from build123d import *

# Parameters (mm, degrees)
BOSS_EXTRUDE1_DEPTH                                  = 30
CBORE_FOR_M5_HEX_HEAD_BOLT1_D                        = 5.5
CBORE_FOR_M5_HEX_HEAD_BOLT1_CBORE_D                  = 12.238
CBORE_FOR_M5_HEX_HEAD_BOLT1_CBORE_DEPTH              = 3.5
CSK_FOR_M4_COUNTERSUNK_RAISED_HEAD_SCREW_D           = 4.3
CSK_FOR_M4_COUNTERSUNK_RAISED_HEAD_SCREW_CSINK_D     = 9.4
CSK_FOR_M4_COUNTERSUNK_RAISED_HEAD_SCREW_CSINK_ANGLE = 90


with BuildPart() as part:
    # Sketch1 → Boss-Extrude1 (new body)
    with BuildSketch(Plane.XY):
        Polygon((0, 0), (0, 40), (120, 40), (120, 30), (10, 30), (10, 0), align=None)
    extrude(amount=BOSS_EXTRUDE1_DEPTH)

    # CBORE for M5 Hex Head Bolt1 (through all)
    with Locations(Plane(origin=(0, 30, 0), x_dir=(-1, 0, 0), z_dir=(0, -1, 0))):
        with Locations((-108, -15.41009868), (-28, -15.41009868)):
            CounterBoreHole(CBORE_FOR_M5_HEX_HEAD_BOLT1_D / 2, CBORE_FOR_M5_HEX_HEAD_BOLT1_CBORE_D / 2, CBORE_FOR_M5_HEX_HEAD_BOLT1_CBORE_DEPTH)

    # CSK for M4 Countersunk Raised Head Screw1 (through all)
    with Locations(Plane(origin=(10, 0, 0), x_dir=(0, 0, -1), z_dir=(1, 0, 0))):
        with Locations((-15.137848296, 12)):
            CounterSinkHole(CSK_FOR_M4_COUNTERSUNK_RAISED_HEAD_SCREW_D / 2, CSK_FOR_M4_COUNTERSUNK_RAISED_HEAD_SCREW_CSINK_D / 2, counter_sink_angle=CSK_FOR_M4_COUNTERSUNK_RAISED_HEAD_SCREW_CSINK_ANGLE)


solid = part.part
Verification items for the finished model (mm, model axes). A direction names the side the tool comes from. Give positions to 0.01 mm unless a question says otherwise; leave off trailing zeros. Write each loop counter-clockwise with the first axis right and the second up, starting at its lowest first coordinate (ties: lowest second). Pieces come first, ordered by that corner, then holes. Notation, with made-up numbers: M 35,61 L 62,61 A14 cw 62,68 Z; hole C 53,47 d6. An arc over 180 degrees is marked long. Write item = value, one per line.
(1) Sectioned sample at D-D (y = 31.5). Record the cut outline in (x, z).
Found:
outline = M 0,0 L 120,0 L 120,30 L 0,30 Z; hole C 28,15.41 d12.24; hole C 108,15.41 d12.24
(2) Go/stop test with flat-tipped pins: pin 1 Ø3.5 at (x, z) = (111, 16.5) entering from -Y; pin 2 Ø7 at (y, z) = (12, 15.14) entering from +X; pin 3 Ø6 at (x, z) = (78, 3.5) entering from -Y. Record where each tip stops, or that it passes through.
Found:
pin_1 = 33.5
pin_2 = 8.8
pin_3 = 30
(3) Access from +Z, -Z, +X, -X, +Y, -Y to the whole of each face (thin tool, end or side, straight path). Record for faces 4 (the face through (120, 35, 15)), 5 (the face through (10, 19, 15)), 6 (the face through (102.164, 31.726, 13.572)).
Found:
face_4 = +Z, -Z, +X, +Y, -Y
face_5 = +Z, -Z, +X, -Y
face_6 = -Y
(4) Sectioned sample at C-C (z = 3.5). Record the cut outline in (x, y).
Found:
outline = M 0,0 L 10,0 L 10,30 L 120,30 L 120,40 L 0,40 Z
(5) Material ranges on line 1 (Z direction, x = 108, y = 37); line 2 (Z direction, x = 108, y = 32); line 3 (Y direction, x = 30, z = 8), recorded low to high.
Found:
line_1 = 0 to 12.66, 18.16 to 30
line_2 = 0 to 9.29, 21.53 to 30
line_3 = 30 to 40
(6) Sectioned sample at A-A (x = 108). Record the cut outline in (y, z).
Found:
outline = M 30,0 L 40,0 L 40,12.66 L 33.5,12.66 L 33.5,9.29 L 30,9.29 Z; M 30,21.53 L 33.5,21.53 L 33.5,18.16 L 40,18.16 L 40,30 L 30,30 Z
(7) Draft check along Y on faces 1 (the face through (25.973, 36.796, 13.552)), 2 (the face through (3.67, 12.09, 12.99)), 3 (the face through (25, 33.5, 17)). Enter one of: released by +Y, released by -Y, zero draft, split by the parting line, or undercut.
Found:
face_1 = zero draft
face_2 = undercut
face_3 = released by -Y
(8) Sectioned sample at B-B (y = 12). Record the cut outline in (x, z).
Found:
outline = M 0,0 L 10,0 L 10,10.44 L 7.45,12.99 L 0,12.99 Z; M 0,17.29 L 7.45,17.29 L 10,19.84 L 10,30 L 0,30 Z
